Model file for the job. Use its own axes, mm. A direction names the side the tool comes from. Give positions to 0.01 mm unless a question says otherwise; leave off trailing zeros. Order: outer loops, then holes, each group sorted by start corner. A loop starts at its lowest first (then second) coordinate and runs counter-clockwise, first axis right, second up. Notation, with made-up numbers: (52.5, -4) - (91.5, -4) arc R22 ccw to (91.5, 27) - close; hole circle Ø5 at (49.25, 17.5). An arc over 180 degrees is marked (long way). Use CSV: the item, a comma, the result in double quotes. Start each with the question number.
(1) Pull direction X, two halves, no side cores. Call faces 1 (the cylindrical face through (-7.493, 0.33, 8.902)), 2 (the flat face through (23, 54, 6)): +X half, -X half, draft (parallel to the pull), parting line (faces both ways), or undercut.
(2) Drop flat-ended pins along their axis: pin 1 Ø4 at (y, z) = (4, 10) entering from -X; pin 2 Ø1.5 at (x, z) = (7, 3) entering from +Y; pin 3 Ø8 at (x, y) = (28, -33) entering from +Z. Give the stop position or say it passes through.
(3) Band-saw the part on D-D, the plane x = -15. Give the cut face in (y, z).
(4) Probe L1, parallel to Y at x = 0, z = 3; L2, parallel to Y at x = 6, z = 5.75; L3, parallel to Z at x = -14, y = 20. List the from-to ranges inside material, lowest first.
(5) Band-saw the part on B-B, the plane x = 0. Give the cut face in (y, z).
(6) Tool access for faces 3 (the flat face through (0, 0, 17)), 4 (the cylindrical face through (2.48, 57.947, 3.972)): list every direction of +Z, -Z, +X, -X, +Y, -Y with a clear straight run to the whole face (end or side of a thin tool).
(7) Band-saw the part on A-A, the plane y = 0. Give the cut face in (x, z).
(8) Band-saw the part on C-C, the plane z = 7.75. Give the cut face in (x, y).
from build123d import *

# Parameters (mm, degrees)
SKETCH_R     = 60
PAD_DEPTH    = 2
PAD001_DEPTH = 5
SKETCH002_R  = 7.5
PAD002_DEPTH = 15
FILLET_R     = 1


with BuildPart() as part:
    # Sketch → Pad (new body)
    with BuildSketch(Plane.XY):
        Circle(SKETCH_R)
    extrude(amount=PAD_DEPTH)

    # Sketch001 → Pad001 (join)
    with BuildSketch(Plane.XY.offset(1)):
        with BuildLine():
            ThreePointArc((5, -57.784081), (0, 58), (-5, -57.784081))
            Line((-5, -57.784081), (-5, -59.791304))
            ThreePointArc((5, -59.791304), (0, 60), (-5, -59.791304))
            Line((5, -57.784081), (5, -59.791304))
        make_face()
    extrude(amount=PAD001_DEPTH)

    # Sketch002 (on Face4 of Pad001) → Pad002 (join)
    with BuildSketch(Plane.XY.offset(2)):
        Circle(SKETCH002_R)
    extrude(amount=PAD002_DEPTH)

    # Fillet
    fillet_edges = [part.edges().sort_by_distance(p)[0] for p in [
        (-7.5, 0, 17),
    ]]
    fillet(fillet_edges, radius=FILLET_R)


solid = part.part
Answer block:
1,face 1,"undercut"
1,face 2,"draft"
2,pin 1,"stops at x = -7.23"
2,pin 2,"stops at y = 59.67"
2,pin 3,"stops at z = 2"
3,outline,"(-58.09, 0) - (58.09, 0) - (58.09, 6) - (56.03, 6) - (56.03, 2) - (-56.03, 2) - (-56.03, 6) - (-58.09, 6) - close"
4,L1,"y = -7.5 to 7.5, 58 to 60"
4,L2,"y = -59.7 to -57.69, -4.5 to 4.5, 57.69 to 59.7"
4,L3,"z = 0 to 2"
5,outline,"(-60, 0) - (60, 0) - (60, 6) - (58, 6) - (58, 2) - (7.5, 2) - (7.5, 16) arc R1 ccw to (6.5, 17) - (-6.5, 17) arc R1 ccw to (-7.5, 16) - (-7.5, 2) - (-60, 2) - close"
6,face 3,"+Z, +X, -X, +Y, -Y"
6,face 4,"+Z"
7,outline,"(-60, 0) - (60, 0) - (60, 6) - (58, 6) - (58, 2) - (7.5, 2) - (7.5, 16) arc R1 ccw to (6.5, 17) - (-6.5, 17) arc R1 ccw to (-7.5, 16) - (-7.5, 2) - (-58, 2) - (-58, 6) - (-60, 6) - close"
8,outline,"circle Ø15 at (0, 0)"
